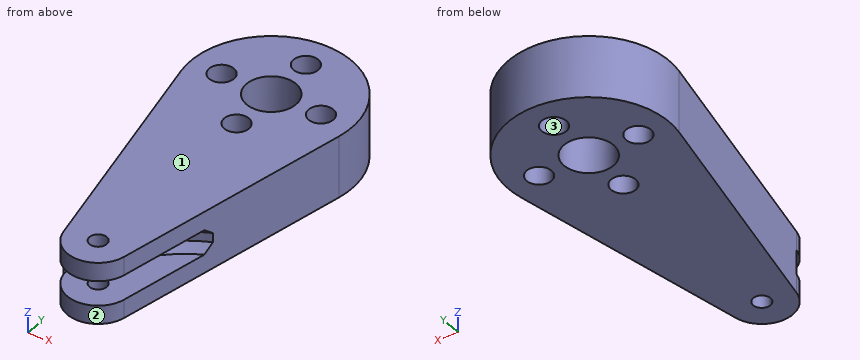
from build123d import *

# Parameters (mm, degrees)
SKETCH1_R                       = 4
SKETCH1_R_2                     = 2
SKETCH1_R_3                     = 1.395
BOSS_EXTRUDE1_DEPTH             = 5
SKETCH2_R                       = 5
BOSS_EXTRUDE2_DEPTH             = 2
BOSS_EXTRUDE3_REACH             = 7
SKETCH3_R                       = 19
BOSS_EXTRUDE3_DIRECTION_2_REACH = 7
CHAMFER1_SIZE                   = 1.25


with BuildPart() as part:
    # Sketch1 → Boss-Extrude1 (new body, symmetric)
    with BuildSketch(Plane.XY):
        with BuildLine():
            Line((4.898582231, -40.924328172), (12.736313801, -2.605054848))
            ThreePointArc((12.736313801, -2.605054848), (0, 13), (-12.736313801, -2.605054848))
            Line((-12.736313801, -2.605054848), (-4.898582231, -40.924328172))
            ThreePointArc((-4.898582231, -40.924328172), (0, -44.922384), (4.898582231, -40.924328172))
        make_face()
        Circle(SKETCH1_R, mode=Mode.SUBTRACT)
        with Locations((0, 8)):
            Circle(SKETCH1_R_2, mode=Mode.SUBTRACT)
        with Locations((8, 0)):
            Circle(SKETCH1_R_2, mode=Mode.SUBTRACT)
        with Locations((0, -8)):
            Circle(SKETCH1_R_2, mode=Mode.SUBTRACT)
        with Locations((-8, 0)):
            Circle(SKETCH1_R_2, mode=Mode.SUBTRACT)
        with Locations((0, -39.922384)):
            Circle(SKETCH1_R_3, mode=Mode.SUBTRACT)
    extrude(amount=BOSS_EXTRUDE1_DEPTH, both=True)


with BuildPart() as body_2:
    # Sketch2 → Boss-Extrude2 (new body, symmetric)
    with BuildSketch(Plane.XY):
        with Locations((0, -39.922384)):
            Circle(SKETCH2_R)
    extrude(amount=BOSS_EXTRUDE2_DEPTH, both=True)


with BuildPart() as part_1:
    add(part.part)

    # Combine1: cut body 2
    add(body_2.part, mode=Mode.SUBTRACT)


with BuildPart() as body_2_2:

    # Boss-Extrude3: up to this face of the body (flat: up to its plane)
    boss_extrude3_end = Plane(part_1.part.faces().sort_by_distance((0, -35.063805356, 2))[0])
    # Sketch3 → Boss-Extrude3 (new body, up to the picked face)
    with BuildSketch(Plane.XY, mode=Mode.PRIVATE) as boss_extrude3_sk1:
        with Locations((15.804791675, -42.49169824)):
            Circle(SKETCH3_R)
    boss_extrude3_tool1 = split(extrude(boss_extrude3_sk1.sketch, amount=BOSS_EXTRUDE3_REACH, mode=Mode.PRIVATE), bisect_by=boss_extrude3_end, keep=Keep.BOTH, mode=Mode.PRIVATE)
    add(boss_extrude3_tool1.solids().sort_by_distance((15.804792, -42.491698, 0))[0])


    # Boss-Extrude3 direction 2: up to this face of the body (flat: up to its plane)
    boss_extrude3_direction_2_end = Plane(part_1.part.faces().sort_by_distance((0, -35.063805356, -2))[0])
    # Sketch3 → Boss-Extrude3 direction 2 (add, up to the picked face)
    with BuildSketch(Plane.XY, mode=Mode.PRIVATE) as boss_extrude3_direction_2_sk1:
        with Locations((15.804791675, -42.49169824)):
            Circle(SKETCH3_R)
    boss_extrude3_direction_2_tool1 = split(extrude(boss_extrude3_direction_2_sk1.sketch, amount=-BOSS_EXTRUDE3_DIRECTION_2_REACH, mode=Mode.PRIVATE), bisect_by=boss_extrude3_direction_2_end, keep=Keep.BOTH, mode=Mode.PRIVATE)
    add(boss_extrude3_direction_2_tool1.solids().sort_by_distance((15.804792, -42.491698, 0))[0])

    # Chamfer1
    chamfer1_edges = [body_2_2.edges().sort_by_distance(p)[0] for p in [
        (-3.195208325, -42.49169824, -2),
        (-3.195208325, -42.49169824, 2),
    ]]
    chamfer(chamfer1_edges, length=CHAMFER1_SIZE)


with BuildPart() as part_2:
    add(part_1.part)

    # Combine2: cut body 2 2
    add(body_2_2.part, mode=Mode.SUBTRACT)


solid = part_2.part
Build history of the part. All positions in model axes, mm. Face numbers are marked on the shaded views. Round coordinates to 2 decimals unless told otherwise and drop trailing zeros. Loops run counter-clockwise (first coordinate to the right, second up) from the corner with the lowest first, then second, coordinate; pieces in that order, holes last. Notation, with made-up numbers: (-8, 34) -> (37, 34) arc R10 ccw to (37, 43) -> close; hole circle Ø4 at (79.5, 10). An arc over 180 degrees is marked (long way). Use CSV: the item, a comma, the result in double quotes. Start each with the question number.
Q1. Saw through at B-B on x = -8. Give the cut face in (y, z).
Q2. Saw through at C-C on z = -3.25. Give the cut face in (x, y) (3 decimals), and give its area (3 significant figures).
Q3. Saw through at A-A on y = -8. Give the cut face in (x, z).
Q4. Saw through at D-D on y = 1. Give the cut face in (x, z), and give its area (3 significant figures).
Q5. Drill centre lines: L1, parallel to Y at x = 0, z = -3.65; L2, parallel to Y at x = 0, z = -0.5; L3, parallel to Z at x = 2.25, y = -38.5. Where is each one in solid material? Low to high.
Q6. Flat gauge pins, fed straight in: pin 1 Ø3 at (x, y) = (8, 0) entering from -Z; pin 2 Ø4 at (x, z) = (7, -2.5) entering from +Y. Where does each tip first touch, or does it go through?
Q7. Mould opens along X. For the marked faces 1, 2 and 3 say: +X half, -X half, draft (parallel to the pull), parting line (faces both ways), or undercut.
Solutions:
1,outline,"(-25.76, -5) -> (-2, -5) -> (-2, 5) -> (-25.76, 5) -> close; (2, -5) -> (10.25, -5) -> (10.25, 5) -> (2, 5) -> close"
2,outline,"(-12.736, -2.605) -> (-4.899, -40.924) arc R5 ccw to (4.899, -40.924) -> (12.736, -2.605) arc R13 ccw (long way) to start; hole circle Ø4 at (-8, 0); hole circle Ø8 at (0, 0); hole circle Ø4 at (0, -8); hole circle Ø4 at (0, 8); hole circle Ø2.79 at (0, -39.922); hole circle Ø4 at (8, 0)"
2,area,"931 mm^2"
3,outline,"(-11.63, -5) -> (-2, -5) -> (-2, 5) -> (-11.63, 5) -> close; (2, -5) -> (11.63, -5) -> (11.63, 5) -> (2, 5) -> close"
4,outline,"(-12.96, -5) -> (-9.73, -5) -> (-9.73, 5) -> (-12.96, 5) -> close; (-6.27, -5) -> (-3.87, -5) -> (-3.87, 5) -> (-6.27, 5) -> close; (3.87, -5) -> (6.27, -5) -> (6.27, 5) -> (3.87, 5) -> close; (9.73, -5) -> (12.96, -5) -> (12.96, 5) -> (9.73, 5) -> close"
4,area,"112 mm^2"
5,L1,"y = -44.92 to -41.32, -38.53 to -10, -6 to -4, 4 to 6, 10 to 13"
5,L2,"y = -31.95 to -10, -6 to -4, 4 to 6, 10 to 13"
5,L3,"z = -5 to -2, 2 to 5"
6,pin 1,"passes through"
6,pin 2,"stops at y = 12"
7,face 1,"draft"
7,face 2,"parting line"
7,face 3,"undercut"
